Geometry: final body of the model. Coordinates: model frame, mm. Coordinates: 2 decimals unless noted, no trailing zeros. Order: outer loops, then holes, each group sorted by start corner. A loop starts at its lowest first (then second) coordinate and runs counter-clockwise, first axis right, second up. Notation, with made-up numbers: (34.5, 14.5) -> (75.5, 14.5) arc R9 cw to (75.5, 19.5) -> close; hole circle Ø4 at (26.25, 56.25). An arc over 180 degrees is marked (long way). Use CSV: the item, a comma, the result in double quotes. Start each with the question number.
from build123d import *

# Parameters (mm, degrees)
EXTRUDE_1_DEPTH     = 6
SKETCH_2_R          = 12.5
CUT_EXTRUDE_1_DEPTH = 153.870315409
CUT_EXTRUDE_2_DEPTH = 153.870315409
SKETCH_6_R          = 2.6
CUT_EXTRUDE_5_DEPTH = 141.247400451
SKETCH_7_R          = 1.6
CUT_EXTRUDE_8_DEPTH = 141.247400451


with BuildPart() as part:
    # 草图1 → 凸台-拉伸1 (new body)
    with BuildSketch(Plane(origin=(0, 0, 0), x_dir=(1, 0, 0), z_dir=(0, 1, 0))):
        Polygon((115.470053838, 0), (57.735026919, 100), (-57.735026919, 100), (-115.470053838, 0), (-57.735026919, -100), (57.735026919, -100), align=None)
    extrude(amount=EXTRUDE_1_DEPTH)

    # 草图2 → 切除-拉伸1 (cut, through all)
    with BuildSketch(Plane(origin=(0, 6, 0), x_dir=(1, 0, 0), z_dir=(0, 1, 0))):
        with Locations(Location((0, 0, 0), (0, 0, 270))):
            Circle(SKETCH_2_R)
    extrude(amount=-CUT_EXTRUDE_1_DEPTH, mode=Mode.SUBTRACT)

    # 草图3 → 切除-拉伸2 (cut, through all)
    with BuildSketch(Plane(origin=(0, 6, 0), x_dir=(1, 0, 0), z_dir=(0, 1, 0))):
        Polygon((-23.094010768, 100), (-98.149545762, -30), (-115.470053838, 0), (-57.735026919, 100), align=None)
        Polygon((98.149545762, -30), (23.094010768, 100), (57.735026919, 100), (115.470053838, 0), align=None)
        Polygon((-75.055534995, -70), (75.055534995, -70), (57.735026919, -100), (-57.735026919, -100), align=None)
    extrude(amount=-CUT_EXTRUDE_2_DEPTH, mode=Mode.SUBTRACT)

    # 草图6 → 切除-拉伸5 (cut, through all)
    with BuildSketch(Plane(origin=(0, 6, 0), x_dir=(1, 0, 0), z_dir=(0, 1, 0))):
        with Locations(Location((-10, -28.284271247, 0), (0, 0, 270))):
            Circle(SKETCH_6_R)
        with Locations(Location((-19.494897428, 22.802389662, 0), (0, 0, 270))):
            Circle(SKETCH_6_R)
        with Locations(Location((29.494897428, 5.481881586, 0), (0, 0, 270))):
            Circle(SKETCH_6_R)
    extrude(amount=-CUT_EXTRUDE_5_DEPTH, mode=Mode.SUBTRACT)

    # 草图7 → 切除-拉伸8 (cut, through all)
    with BuildSketch(Plane(origin=(0, 0, 0), x_dir=(1, 0, 0), z_dir=(0, 1, 0))):
        with Locations(Location((60, -32.5, 0), (0, 0, 270))):
            Circle(SKETCH_7_R)
        with Locations(Location((28, -32.5, 0), (0, 0, 270))):
            Circle(SKETCH_7_R)
        with Locations(Location((60, -57.5, 0), (0, 0, 270))):
            Circle(SKETCH_7_R)
        with Locations(Location((28, -57.5, 0), (0, 0, 270))):
            Circle(SKETCH_7_R)
        with Locations(Location((-58.145825623, -35.711524227, 0), (0, 0, 270))):
            Circle(SKETCH_7_R)
        with Locations(Location((-42.145825623, -7.998711306, 0), (0, 0, 270))):
            Circle(SKETCH_7_R)
        with Locations(Location((-79.796460718, -23.211524227, 0), (0, 0, 270))):
            Circle(SKETCH_7_R)
        with Locations(Location((-63.796460718, 4.501288694, 0), (0, 0, 270))):
            Circle(SKETCH_7_R)
        with Locations(Location((-1.854174377, 68.211524227, 0), (0, 0, 270))):
            Circle(SKETCH_7_R)
        with Locations(Location((14.145825623, 40.498711306, 0), (0, 0, 270))):
            Circle(SKETCH_7_R)
        with Locations(Location((19.796460718, 80.711524227, 0), (0, 0, 270))):
            Circle(SKETCH_7_R)
        with Locations(Location((35.796460718, 52.998711306, 0), (0, 0, 270))):
            Circle(SKETCH_7_R)
    extrude(amount=CUT_EXTRUDE_8_DEPTH, mode=Mode.SUBTRACT)


solid = part.part
(1) Mould query, pull axis Z, two halves, no side actions, for faces 1 (the face through (0, 3, -100)), 2 (the face through (26.957, 3.042, -6.046)), 3 (the face through (-1, 3, 70)). Classes: pulls with the +Z half, pulls with the -Z half, needs draft (parallel to the pull), parting line crosses it, or undercut.
(2) Section B-B (x = -25.5). Return loops of the section in (y, z).
(3) Line query: line 1 (Z direction, x = -20, y = 2.95); line 2 (X direction, y = 4.3, z = 57.5); line 3 (Z direction, x = -8.5, y = 2.6). Output: solid intervals per line, ascending. Write a range as from..to.
(4) Section A-A (y = 4.45). State how many separate pieces and enclosed holes the cut face has, then the cut area to 3 significant figures.
(5) First-contact query: pin 1 (5 mm diameter, centred on x = 19.8, z = -80.71, fed in from +Y); pin 2 (2 mm diameter, centred on y = 2.5, z = 5, fed in from +X); pin 3 (2.5 mm diameter, centred on x = 60, z = 57.5, fed in from +Y). Flat tips, straight axial feed; report the tip coordinate or a pass-through.
(6) Section C-C (z = 42). Return loops of the section in (x, y).
Check sheet entries:
1,face 1,"pulls with the -Z half"
1,face 2,"undercut"
1,face 3,"pulls with the +Z half"
2,outline,"(0, -95.83) -> (6, -95.83) -> (6, 70) -> (0, 70) -> close"
3,line 1,"z = -100..-25.35, -20.25..70"
3,line 2,"x = -82.27..26.4, 29.6..58.4, 61.6..82.27"
3,line 3,"z = -100..-9.17, 9.17..26.16, 30.41..70"
4,separate pieces,"1"
4,enclosed holes,"16"
4,area,"22,000 mm^2"
5,pin 1,"stops at y = 6"
5,pin 2,"stops at x = 84.29"
5,pin 3,"passes through"
6,outline,"(-91.22, 0) -> (91.22, 0) -> (91.22, 6) -> (-91.22, 6) -> close"
